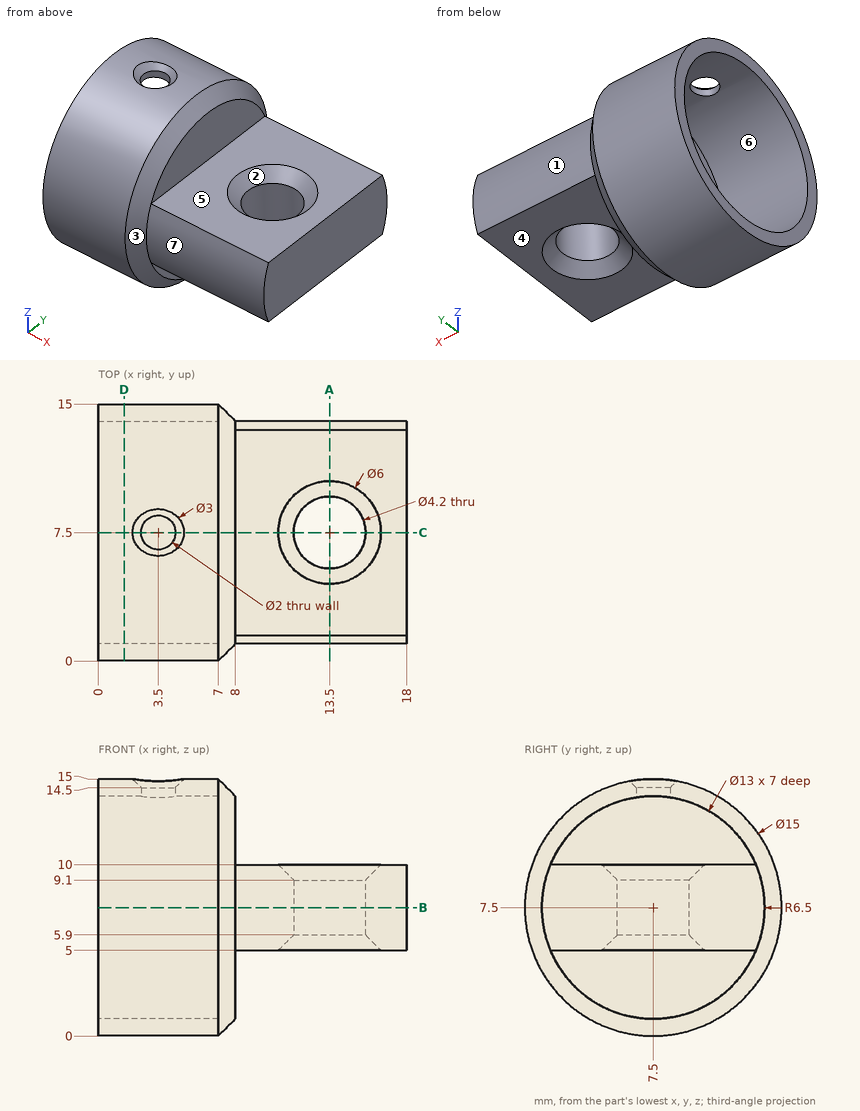
Source: three-view drawing plus pictorial views. Frame: mm from the lowest corner of the part. A direction names the side the tool comes from. Round coordinates to 2 decimals unless told otherwise and drop trailing zeros. Write each loop counter-clockwise with the first axis right and the second up, starting at its lowest first coordinate (ties: lowest second). Pieces come first, ordered by that corner, then holes. Notation, with made-up numbers: M 36,3.5 L 43,3.5 A19 cw 43,32.5 Z; hole C 14,27 d11. An arc over 180 degrees is marked long. Use CSV: the item, a comma, the result in double quotes. Start each with the question number.
Q1. Access query for the marked faces 4, 5, 6 and 7. Directions: +Z, -Z, +X, -X, +Y, -Y. A direction counts if a zero-diameter tool reaches every point of the face in a straight line with its end or side. Return the directions, or none.
Q2. Cut plane C-C on y = 7.5. Output: boundary loops of the cut face in (x, z).
Q3. Cut plane A-A on x = 13.5. Output: boundary loops of the cut face in (y, z), plus the area to 3 significant figures.
Q4. Cut plane D-D on x = 1.5. Output: boundary loops of the cut face in (y, z).
Q5. Pull-direction query (X, two-part tool) for the marked faces 1, 2 and 3; classes: +X half, -X half, draft (parallel to the pull), parting line (faces both ways), or undercut.
Q6. Cut plane B-B on z = 7.5. Output: boundary loops of the cut face in (x, y), plus the area to 3 significant figures.
Q7. Line query: line 1 (Z direction, x = 5.5, y = 7.5); line 2 (X direction, y = 12.75, z = 7); line 3 (X direction, y = 9.5, z = 12.5). Output: solid intervals per line, ascending. Write a range as from..to.
Q8. First-contact query: P1, Ø3, axis at y = 6, z = 12, coming from the +X side; P2, Ø3, axis at x = 8.5, y = 10, coming from the -Z side; P3, Ø8, axis at x = 13.5, y = 12.5, coming from the +Z side. Flat tips, straight axial feed; report the tip coordinate or a pass-through.
Results found:
1,face 4,"-Z, +X, +Y, -Y"
1,face 5,"+Z, +X, +Y, -Y"
1,face 6,"-X"
1,face 7,"+X, -Y"
2,outline,"M 0,0 L 7,0 L 8,1 L 8,5 L 10.5,5 L 11.4,5.9 L 11.4,9.1 L 10.5,10 L 8,10 L 8,14 L 7,15 L 5,15 L 4.5,14.5 L 4.5,14 L 7,14 L 7,1 L 0,1 Z; M 0,14 L 2.5,14 L 2.5,14.5 L 2,15 L 0,15 Z; M 15.6,5.9 L 16.5,5 L 18,5 L 18,10 L 16.5,10 L 15.6,9.1 Z"
3,outline,"M 1.5,5 L 4.5,5 L 5.4,5.9 L 5.4,9.1 L 4.5,10 L 1.5,10 A6.5 ccw Z; M 9.6,5.9 L 10.5,5 L 13.5,5 A6.5 ccw 13.5,10 L 10.5,10 L 9.6,9.1 Z"
3,area,"40.7 mm^2"
4,outline,"C 7.5,7.5 d15; hole C 7.5,7.5 d13"
5,face 1,"draft"
5,face 2,"undercut"
5,face 3,"+X half"
6,outline,"M 0,0 L 7,0 L 8,1 L 18,1 L 18,14 L 8,14 L 7,15 L 0,15 L 0,14 L 7,14 L 7,1 L 0,1 Z; hole C 13.5,7.5 d4.2"
6,area,"144 mm^2"
7,line 1,"0..1, 14..15"
7,line 2,"7..18"
7,line 3,"7..8"
8,P1,"x = 8"
8,P2,"z = 0.36"
8,P3,"z = 10"
